```python
from build123d import *

# Parameters (mm, degrees)
SKETCH1_R           = 6.35
BOSS_EXTRUDE1_DEPTH = 12.7
CUT_EXTRUDE2_DEPTH  = 13.7
FILLET1_R           = 12.7
SKETCH4_R           = 12.7
SKETCH4_R_2         = 6.35
BOSS_EXTRUDE2_DEPTH = 6.35
SKETCH2_W           = 27.073872012
SKETCH2_H           = 29.596885175
CUT_EXTRUDE1_DEPTH  = 9.525


with BuildPart() as part:
    # Sketch1 → Boss-Extrude1 (new body)
    with BuildSketch(Plane(origin=(0, 0, 0), x_dir=(1, 0, 0), z_dir=(0, 1, 0))):
        with BuildLine():
            Line((1.339902706, -174.625), (-42.399739587, -174.625))
            ThreePointArc((-42.399739587, -174.625), (-50.754602331, -177.79991886), (-59.131949668, -174.684811669))
            Line((-59.131949668, -174.684811669), (-96.253765638, -142.415309363))
            ThreePointArc((-96.253765638, -142.415309363), (-144.617963608, -71.634466036), (-152.13989844, 13.761341376))
            ThreePointArc((-152.13989844, 13.761341376), (-145.072520944, 18.99854995), (-139.553151074, 12.149262793))
            ThreePointArc((-139.553151074, 12.149262793), (-129.869632709, -52.503000495), (-91.90140484, -105.720472707))
            Line((-91.90140484, -105.720472707), (-48.88478864, -143.114246675))
            ThreePointArc((-48.88478864, -143.114246675), (-33.347524936, -152.357947214), (-15.556989968, -155.575))
            Line((-15.556989968, -155.575), (1.339902706, -155.575))
            ThreePointArc((1.339902706, -155.575), (10.864902706, -165.1), (1.339902706, -174.625))
        make_face()
        with Locations((-50.8, -165.1)):
            Circle(SKETCH1_R, mode=Mode.SUBTRACT)
        with BuildLine():
            Line((0, -161.925), (1.339902706, -161.925))
            ThreePointArc((1.339902706, -161.925), (4.514902706, -165.1), (1.339902706, -168.275))
            Line((1.339902706, -168.275), (0, -168.275))
            ThreePointArc((0, -168.275), (-3.175, -165.1), (0, -161.925))
        make_face(mode=Mode.SUBTRACT)
    extrude(amount=BOSS_EXTRUDE1_DEPTH)

    # Sketch3 → Cut-Extrude2 (cut, through all)
    with BuildSketch(Plane(origin=(0, 12.7, 0), x_dir=(1, 0, 0), z_dir=(0, 1, 0))):
        with BuildLine():
            Line((-64.278893585, -138.146187914), (-96.067379674, -110.512878542))
            ThreePointArc((-96.067379674, -110.512878542), (-104.093661598, -102.988093371), (-111.532318829, -94.88192461))
            ThreePointArc((-111.532318829, -94.88192461), (-120.588765116, -93.847414192), (-122.222718656, -102.815113283))
            ThreePointArc((-122.222718656, -102.815113283), (-108.389889378, -121.287896312), (-92.087790804, -137.622903528))
            Line((-92.087790804, -137.622903528), (-75.989121055, -151.617263638))
            ThreePointArc((-75.989121055, -151.617263638), (-63.398469458, -150.736839511), (-64.278893585, -138.146187914))
        make_face()
        with BuildLine():
            ThreePointArc((-122.168303836, -80.727586976), (-124.013598755, -88.474110491), (-131.62448434, -86.131428157))
            ThreePointArc((-131.62448434, -86.131428157), (-143.140144863, -54.755391727), (-148.016867664, -21.690551276))
            ThreePointArc((-148.016867664, -21.690551276), (-146.581764091, -20.040770563), (-144.860415421, -21.389198324))
            ThreePointArc((-144.860415421, -21.389198324), (-136.771142128, -52.303847297), (-122.168303836, -80.727586976))
        make_face()
    extrude(amount=-CUT_EXTRUDE2_DEPTH, mode=Mode.SUBTRACT)

    # Fillet1
    fillet1_edges = [part.edges().sort_by_distance(p)[0] for p in [
        (-42.399739587, 6.35, 174.625),
    ]]
    fillet(fillet1_edges, radius=FILLET1_R)

    # Sketch4 → Boss-Extrude2 (add)
    with BuildSketch(Plane(origin=(0, 0, 0), x_dir=(1, 0, 0), z_dir=(0, 1, 0))):
        with Locations((-50.8, -165.1)):
            Circle(SKETCH4_R)
        with Locations((-50.8, -165.1)):
            Circle(SKETCH4_R_2, mode=Mode.SUBTRACT)
        with BuildLine():
            Line((1.339902706, -174.625), (-15.556989968, -174.625))
            ThreePointArc((-15.556989968, -174.625), (-25.081989968, -165.1), (-15.556989968, -155.575))
            Line((-15.556989968, -155.575), (1.339902706, -155.575))
            ThreePointArc((1.339902706, -155.575), (10.864902706, -165.1), (1.339902706, -174.625))
        make_face()
        with BuildLine():
            Line((1.339902706, -161.925), (0, -161.925))
            ThreePointArc((0, -161.925), (-3.175, -165.1), (0, -168.275))
            Line((0, -168.275), (1.339902706, -168.275))
            ThreePointArc((1.339902706, -168.275), (4.514902706, -165.1), (1.339902706, -161.925))
        make_face(mode=Mode.SUBTRACT)
    extrude(amount=-BOSS_EXTRUDE2_DEPTH)

    # Sketch2 → Cut-Extrude1 (cut)
    with BuildSketch(Plane(origin=(0, 12.7, 0), x_dir=(1, 0, 0), z_dir=(0, 1, 0))):
        with Locations((4.011936006, -165.256904056)):
            Rectangle(SKETCH2_W, SKETCH2_H)
    extrude(amount=-CUT_EXTRUDE1_DEPTH, mode=Mode.SUBTRACT)


solid = part.part
```
For this review, take the finished solid that the model builds, in its own axes (mm). A direction names the side the tool comes from. Round coordinates to 2 decimals unless told otherwise and drop trailing zeros. Write each loop counter-clockwise with the first axis right and the second up, starting at its lowest first coordinate (ties: lowest second). Pieces come first, ordered by that corner, then holes.
1) Take a section at B-B on z = 114.5. Give the boundary of the cut face in (x, y), then the cut area to 3 significant figures.
Answer below:
outline: (-121.9, 0) - (-113.95, 0) - (-113.95, 12.7) - (-121.9, 12.7) - close; (-91.48, 0) - (-81.8, 0) - (-81.8, 12.7) - (-91.48, 12.7) - close
area: 224 mm2
2) Machinability: for faces 5 (the face through (-84.151, 6.439, 144.522)), 6 (the face through (-18, 3, 174.625)), 7 (the face through (-70.69, 6.26, 124.16)), which of the approach directions +Z, -Z, +X, -X, +Y, -Y give a long, thin tool a straight path to every point of the face, cutting with its end or side? Answer none if there is none.
Answer below:
face 5: +Y, -Y
face 6: +Z, +X, +Y, -Y
face 7: -Z, +X, +Y, -Y
3) Insertion check: pin 1 Ø9.5 at (x, y) = (-26, 5.5) entering from +Z (3 decimals); pin 2 Ø10 at (x, z) = (-50.8, 165.1) entering from -Y; pin 3 Ø1.9 at (x, y) = (-10, -2.5) entering from -Z (3 decimals); pin 4 Ø4 at (x, y) = (-61, 7) entering from -Z. Each pin has a flat end and moves straight along its axis. Give the tip position at first contact, or say it passes through.
Answer below:
pin 1: stops at z = 174.625
pin 2: passes through
pin 3: stops at z = 155.575
pin 4: stops at z = 130.84
4) Take a section at D-D on z = 165.1. Give the boundary of the cut face in (x, y) (3 decimals), then the cut area to 3 significant figures.
Answer below:
outline: (-70.158, 0) - (-63.5, 0) - (-63.5, -6.35) - (-57.15, -6.35) - (-57.15, 12.7) - (-70.158, 12.7) - close; (-44.45, -6.35) - (-38.1, -6.35) - (-38.1, 0) - (-25.082, 0) - (-25.082, -6.35) - (-3.175, -6.35) - (-3.175, 3.175) - (-9.525, 3.175) - (-9.525, 12.7) - (-44.45, 12.7) - close; (4.515, -6.35) - (10.865, -6.35) - (10.865, 3.175) - (4.515, 3.175) - close
area: 909 mm2
5) Take a section at C-C on x = -105.5. Give the boundary of the cut face in (y, z), then the cut area to 3 significant figures.
Answer below:
outline: (0, 92.15) - (12.7, 92.15) - (12.7, 101.55) - (0, 101.55) - close; (0, 124.54) - (12.7, 124.54) - (12.7, 133.75) - (0, 133.75) - close
area: 236 mm2
6) For line 1 along X through (y, z) = (-4.5, 165.1) (3 decimals); line 2 along Z through (x, y) = (-50.8, -2.25); line 3 along Y through (x, z) = (-89.5, 115), list the stretches that pass through material, from the lowest coordinate up.
Answer below:
line 1: x = -63.5 to -57.15, -44.45 to -38.1, -25.082 to -3.175, 4.515 to 10.865
line 2: z = 152.4 to 158.75, 171.45 to 177.8
line 3: y = 0 to 12.7
7) Mouldability with a two-part tool opening along Z and no side actions: class faces 1 (the face through (-33.586, 6.261, 152.268)), 2 (the face through (-9.525, 8, 165)), 3 (the face through (-123.906, 6.439, 88.411)), 4 (the face through (-77.43, 6.26, 158.78)) as +Z half, -Z half, draft (parallel to the pull), parting line (faces both ways), or undercut.
Answer below:
face 1: -Z half
face 2: draft
face 3: undercut
face 4: +Z half
8) Take a section at A-A on y = -3.5. Give the boundary of the cut face in (x, z) (3 decimals), then the cut area to 3 significant figures.
Answer below:
outline: circle Ø25.4 at (-50.8, 165.1); (-15.557, 155.575) - (1.34, 155.575) arc R9.525 ccw to (1.34, 174.625) - (-15.557, 174.625) arc R9.525 ccw to start; hole circle Ø12.7 at (-50.8, 165.1); hole (0, 161.925) - (1.34, 161.925) arc R3.175 ccw to (1.34, 168.275) - (0, 168.275) arc R3.175 ccw to start
area: 947 mm2
